Geometry check sheet. Reference: the model listing, model coordinates, mm. Face numbers are marked on the shaded views. A direction names the side the tool comes from. Coordinates: 2 decimals unless noted, no trailing zeros. Write each loop counter-clockwise with the first axis right and the second up, starting at its lowest first coordinate (ties: lowest second). Pieces come first, ordered by that corner, then holes.
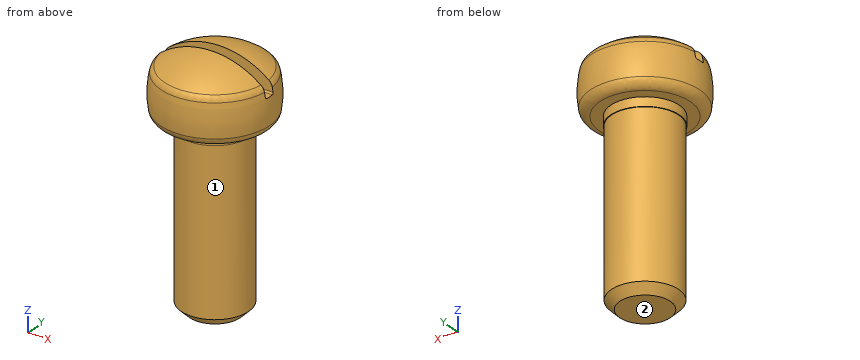
from build123d import *

# Parameters (mm, degrees)
CUT_EXTRUDE1_DEPTH      = 21.516664352
CUT_EXTRUDE1_DEPTH_BACK = 21.516664352
SKETCH9_W               = 4.05765
SKETCH9_H               = 1.57988
FILLET1_R               = 0.225425
FILLET2_R               = 1.35255


with BuildPart() as part:
    # Sketch2 → Revolve1 (revolve)
    with BuildSketch(Plane(origin=(0, 0, 0), x_dir=(0, 0, -1), z_dir=(1, 0, 0)), mode=Mode.PRIVATE) as revolve1_sk:
        with BuildLine():
            Line((-8.1915, 7.50443), (-8.1915, 4.85775))
            Line((-8.1915, 4.85775), (-6.9215, 4.85775))
            Line((-6.9215, 4.85775), (-6.9215, 4.7625))
            Line((-6.9215, 4.7625), (16.017875, 4.7625))
            Line((16.017875, 4.7625), (17.2085, 3.571875))
            Line((17.2085, 3.571875), (17.2085, 0))
            Line((17.2085, 0), (-17.2085, 0))
            ThreePointArc((-17.2085, 0), (-16.511577735, 3.988547218), (-14.5034, 7.50443))
            ThreePointArc((-14.5034, 7.50443), (-11.34745, 7.8994), (-8.1915, 7.50443))
        make_face()
    revolve(revolve1_sk.sketch.rotate(Axis((0, 0, 17.2085), (0, 0, -1)), 90), axis=Axis((0, 0, 17.2085), (0, 0, -1)))

    # Sketch9 → Cut-Extrude1 (cut, two sides: drawn at the far end of the back side and taken through both)
    with BuildSketch(Plane(origin=(0, 0, 0), x_dir=(0, 0, -1), z_dir=(1, 0, 0)).offset(-CUT_EXTRUDE1_DEPTH_BACK)):
        with Locations((-15.179675, 0)):
            Rectangle(SKETCH9_W, SKETCH9_H)
    extrude(amount=CUT_EXTRUDE1_DEPTH + CUT_EXTRUDE1_DEPTH_BACK, mode=Mode.SUBTRACT)

    # Fillet1
    fillet1_edges = [part.edges().sort_by_distance(p)[0] for p in [
        (0, 0.78994, 13.15085),
        (0, -0.78994, 13.15085),
    ]]
    fillet(fillet1_edges, radius=FILLET1_R)

    # Fillet2
    fillet2_edges = [part.edges().sort_by_distance(p)[0] for p in [
        (-7.50443, 0, 8.1915),
        (0, -7.50443, 14.5034),
        (0, 7.50443, 14.5034),
    ]]
    fillet(fillet2_edges, radius=FILLET2_R)


solid = part.part
1. Access from +Z, -Z, +X, -X, +Y, -Y to the whole of each face (thin tool, end or side, straight path). Record for the marked faces 1 and 2.
Computed values:
face 1: -Z
face 2: -Z, +X, -X, +Y, -Y
2. Gauge pin test, flat ends, axial feed: pin 1 Ø8 at (x, y) = (-4, -5) entering from +Z; pin 2 Ø8 at (y, z) = (3, -1) entering from -X; pin 3 Ø3 at (y, z) = (3.5, 4.5) entering from +X. Record the tip position at first contact, or that the pin passes through.
Computed values:
pin 1: stops at z = 16.96
pin 2: stops at x = -4.76
pin 3: stops at x = 4.32
3. Thickness scan on line 1 along Z through (x, y) = (2.25, -0.5); line 2 along Y through (x, z) = (2.25, 11.5); line 3 along Z through (x, y) = (-6, -0.5). Record the ranges inside material, lowest first.
Computed values:
line 1: z = -17.21 to 13.15
line 2: y = -7.57 to 7.57
line 3: z = 8.19 to 13.15
4. Sectioned sample at A-A, the plane z = -1.5. Record the boundary of the cut face in (x, y) (1 decimal), and give its area (3 significant figures).
Computed values:
outline: circle Ø9.5 at (0, 0)
area: 71.3 mm2
